Drawing for the job (mm, zero at the part's lowest x, y, z). Give positions to 0.01 mm unless a question says otherwise; leave off trailing zeros. Loops run counter-clockwise (first coordinate to the right, second up) from the corner with the lowest first, then second, coordinate; pieces in that order, holes last. Notation, with made-up numbers: (24.25, 58) -> (47.25, 58) arc R21 cw to (47.25, 91) -> close; hole circle Ø8 at (78, -31). An arc over 180 degrees is marked (long way). Use CSV: the item, a comma, the result in double quotes. Start each with the question number.
(1) Cut at A-A on x = 16. Write the cut outline in (y, z), then the cut area to 3 significant figures.
(2) Cut at B-B on z = 7.75. Write the cut outline in (x, y), then the cut area to 3 significant figures.
(3) Cut at C-C on y = 24.5. Write the cut outline in (x, z).
(4) Drill centre lines: probe 1 along Y at (x, z) = (16, 3.75); probe 2 along Y at (x, z) = (6, 7.5); probe 3 along X at (y, z) = (27.5, 6.5). Where is each one in solid material? Low to high.
(5) Pull direction Y, two halves, no side cores. Call the marked faces 1, 2, 3 and 4: pulls with the +Y half, pulls with the -Y half, needs draft (parallel to the pull), parting line crosses it, or undercut.
(6) Cut at D-D on x = 3. Write the cut outline in (y, z).
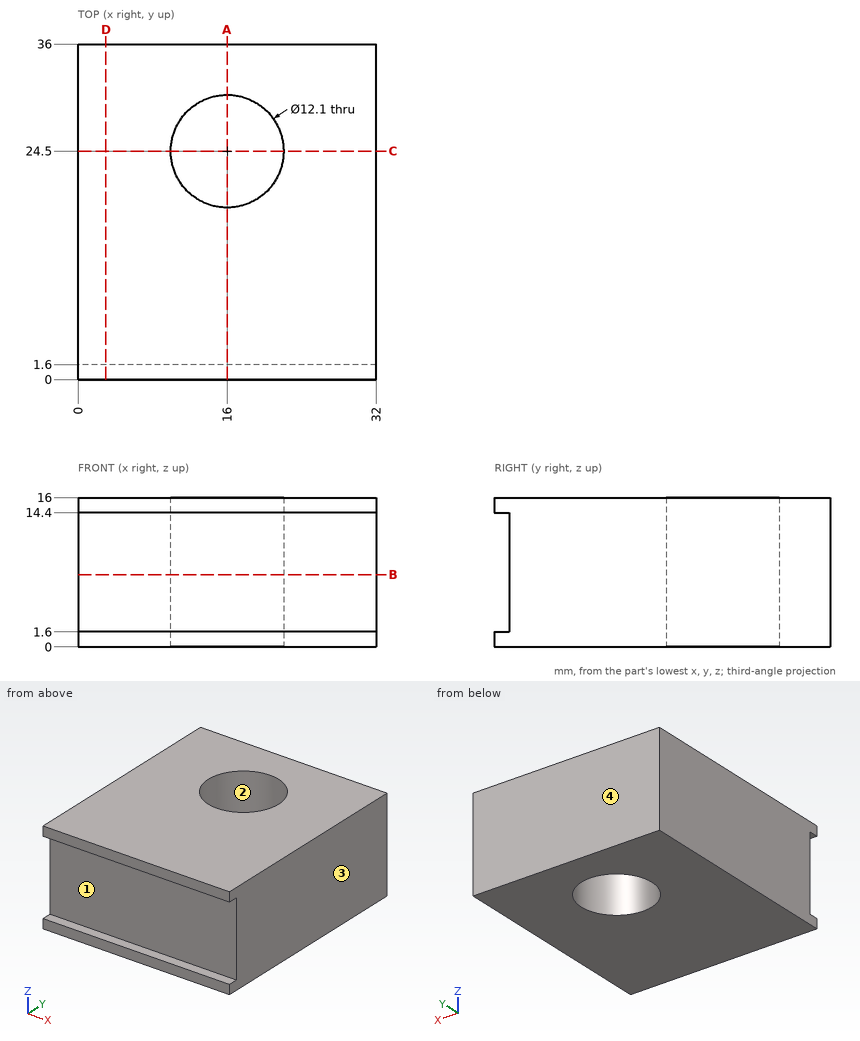
Check result:
1,outline,"(0, 0) -> (18.45, 0) -> (18.45, 16) -> (0, 16) -> (0, 14.4) -> (1.6, 14.4) -> (1.6, 1.6) -> (0, 1.6) -> close; (30.55, 0) -> (36, 0) -> (36, 16) -> (30.55, 16) -> close"
1,area,"362 mm²"
2,outline,"(0, 1.6) -> (32, 1.6) -> (32, 36) -> (0, 36) -> close; hole circle Ø12.1 at (16, 24.5)"
2,area,"986 mm²"
3,outline,"(0, 0) -> (9.95, 0) -> (9.95, 16) -> (0, 16) -> close; (22.05, 0) -> (32, 0) -> (32, 16) -> (22.05, 16) -> close"
4,probe 1,"1.6 to 18.45, 30.55 to 36"
4,probe 2,"1.6 to 36"
4,probe 3,"0 to 10.75, 21.25 to 32"
5,face 1,"pulls with the -Y half"
5,face 2,"undercut"
5,face 3,"needs draft"
5,face 4,"pulls with the +Y half"
6,outline,"(0, 0) -> (36, 0) -> (36, 16) -> (0, 16) -> (0, 14.4) -> (1.6, 14.4) -> (1.6, 1.6) -> (0, 1.6) -> close"
